Can you work these out from the drawing? Everything is in mm from the part's minimum corner. Round coordinates to 2 decimals unless told otherwise and drop trailing zeros. Order: outer loops, then holes, each group sorted by start corner. A loop starts at its lowest first (then second) coordinate and runs counter-clockwise, first axis right, second up. Notation, with made-up numbers: M 35.25,49.25 L 49.25,49.25 A8 ccw 49.25,56.25 Z; hole C 70.5,9 d8. An arc over 180 degrees is marked long. Write each question's results on one line, items separated by ' | '. Start each with the question number.
1. Suppose I cut it at A-A on x = 10. Write out the boundary of the cut face in (y, z) (1 decimal), and give its area (3 significant figures).
2. Suppose I cut it at B-B on y = 3.75. Give the number of separate pieces and of enclosed holes in the cut face, and give its area (3 significant figures).
3. Suppose I cut it at C-C on z = 7. Write out the boundary of the cut face in (x, y) (1 decimal), and give its area (3 significant figures).
4. Please list where these lines run through material, in increasing order: L1, parallel to X at y = 5.75, z = 10 (1 decimal); L2, parallel to Z at x = 11, y = 8.5.
5. I'm going to push a flat-ended pin straight in: pin 1 (2 mm diameter, centred on x = 30.5, z = 31.5, fed in from +Y). Where does the tip first touch, or does it pass through?
6. Suppose I cut it at D-D on x = 31. Write out the boundary of the cut face in (y, z) (1 decimal).
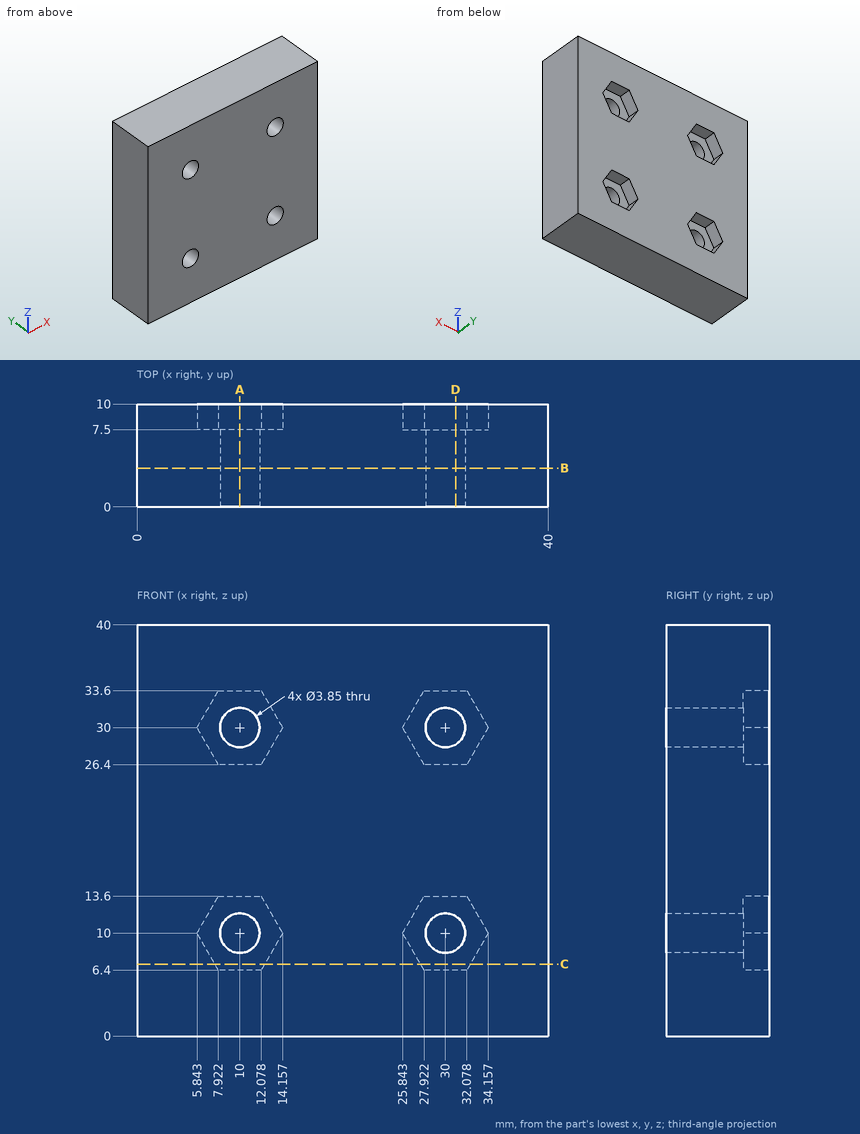
Filled sheet:
1) outline: M 0,0 L 10,0 L 10,6.4 L 7.5,6.4 L 7.5,8.1 L 0,8.1 Z; M 0,11.9 L 7.5,11.9 L 7.5,13.6 L 10,13.6 L 10,26.4 L 7.5,26.4 L 7.5,28.1 L 0,28.1 Z; M 0,31.9 L 7.5,31.9 L 7.5,33.6 L 10,33.6 L 10,40 L 0,40 Z | area: 306 mm^2
2) separate pieces: 1 | enclosed holes: 4 | area: 1,550 mm^2
3) outline: M 0,0 L 40,0 L 40,10 L 32.4,10 L 32.4,7.5 L 27.6,7.5 L 27.6,10 L 12.4,10 L 12.4,7.5 L 7.6,7.5 L 7.6,10 L 0,10 Z | area: 376 mm^2
4) L1: x = 0 to 8.1, 11.9 to 28.1, 31.9 to 40 | L2: z = 0 to 6.4, 13.6 to 26.4, 33.6 to 40
5) pin 1: stops at y = 7.5
6) outline: M 0,0 L 10,0 L 10,6.4 L 7.5,6.4 L 7.5,8.4 L 0,8.4 Z; M 0,11.6 L 7.5,11.6 L 7.5,13.6 L 10,13.6 L 10,26.4 L 7.5,26.4 L 7.5,28.4 L 0,28.4 Z; M 0,31.6 L 7.5,31.6 L 7.5,33.6 L 10,33.6 L 10,40 L 0,40 Z
